Verification items for this drawing (mm, ordinates from the low corner). A direction names the side the tool comes from. Round coordinates to 2 decimals unless told otherwise and drop trailing zeros. Order: outer loops, then holes, each group sorted by start corner. A loop starts at its lowest first (then second) coordinate and runs counter-clockwise, first axis right, second up. Notation, with made-up numbers: (-30, 35) -> (-20, 35) arc R14 ccw to (-20, 48) -> close; hole circle Ø7 at (43, 39). An arc over 180 degrees is marked (long way). Answer in a Markdown table with one row per item. Add a question column.
1. Sectioned sample at A-A, the plane y = 5.5. Record the boundary of the cut face in (x, z), then the cut area to 3 significant figures.
2. Material ranges on L1, parallel to X at y = 19, z = 4; L2, parallel to Y at x = 19.05, z = 8.75; L3, parallel to Y at x = 438.15, z = 25 (3 decimals), recorded low to high. Write a range as from..to.
3. Sectioned sample at B-B, the plane z = 39. Count the separate pieces of the cut face and the enclosed holes in it, then the cut area to 3 significant figures.
4. Access from +Z, -Z, +X, -X, +Y, -Y to the whole of each face (thin tool, end or side, straight path). Record for the marked faces 1 and 2.
5. Depth check by flat-ended pin: P1, Ø10, axis at x = 439, y = 19.5, coming from the -Z side; P2, Ø11.5, axis at x = 506.5, y = 20, coming from the +Z side; P3, Ø3, axis at y = 28.5, z = 18.5, coming from the +X side. Enter the tip coordinate at first touch or a pass-through.
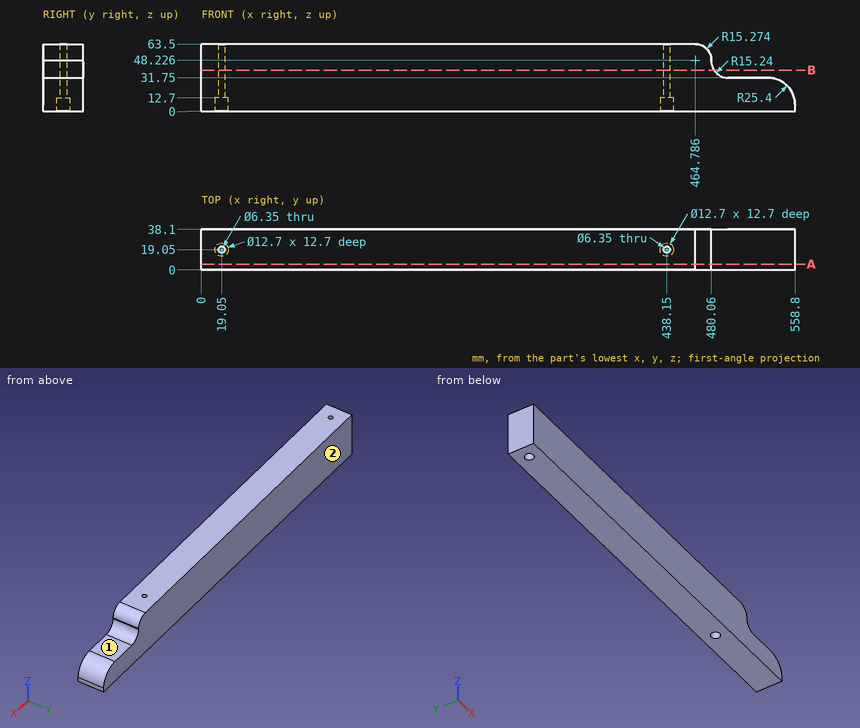
Answer key:
| question | item | result |
|---|---|---|
| 1 | outline | (0, 0) -> (558.8, 0) -> (558.8, 6.35) arc R25.4 ccw to (533.4, 31.75) -> (495.3, 31.75) arc R15.24 cw to (480.06, 46.99) -> (480.06, 48.26) arc R15.27 ccw to (464.82, 63.5) -> (0, 63.5) -> close |
| 1 | area | 32,800 mm² |
| 2 | L1 | x = 0..12.7, 25.4..431.8, 444.5..558.8 |
| 2 | L2 | y = 0..12.7, 25.4..38.1 |
| 2 | L3 | y = 0..15.875, 22.225..38.1 |
| 3 | separate pieces | 1 |
| 3 | enclosed holes | 2 |
| 3 | area | 18,300 mm² |
| 4 | face 1 | +Z, +X, +Y, -Y |
| 4 | face 2 | +Z, -Z, +X, -X, +Y |
| 5 | P1 | stops at z = 12.7 |
| 5 | P2 | stops at z = 31.75 |
| 5 | P3 | stops at x = 556.46 |
